Read the model definition and answer for the solid it produces. Units are mm, in the model's axes. A direction names the side the tool comes from. Coordinates: 2 decimals unless noted, no trailing zeros. Order: outer loops, then holes, each group sorted by start corner. A loop starts at its lowest first (then second) coordinate and runs counter-clockwise, first axis right, second up. Notation, with made-up numbers: (13, 6.5) -> (65, 6.5) arc R18 cw to (65, 11.5) -> close; hole circle Ø3 at (86.25, 19.25). An arc over 180 degrees is marked (long way). Use CSV: the item, a comma, the result in double quotes.
```python
from build123d import *

# Parameters (mm, degrees)
EXTRUDE_1_DEPTH          = 20
SKETCH_2_R               = 4.5
CUT_EXTRUDE_2_DEPTH      = 95.074438611
MIRROR_2_COPY_1_SKETCH_R = 4.5
MIRROR_2_COPY_1_DEPTH    = 95.074438611
SKETCH_3_R               = 55
CUT_EXTRUDE_3_DEPTH      = 95.074438611
EXTRUDE_2_DEPTH          = 20
SKETCH_6_R               = 5
CUT_EXTRUDE_4_DEPTH      = 143.828568571
SKETCH_1312_R            = 2.5
CUT_EXTRUDE_5_DEPTH      = 10


with BuildPart() as part:
    # 草圖1 → 填料-伸長1 (new body)
    with BuildSketch(Plane.XY):
        with BuildLine():
            Line((-55, 65), (55, 65))
            ThreePointArc((55, 65), (62.071067812, 62.071067812), (65, 55))
            Line((65, 55), (65, -65))
            Line((65, -65), (-65, -65))
            Line((-65, -65), (-65, 55))
            ThreePointArc((-65, 55), (-62.071067812, 62.071067812), (-55, 65))
        make_face()
    extrude(amount=EXTRUDE_1_DEPTH)

    # 草圖2 → 除料-伸長2 (cut, through all)
    with BuildSketch(Plane.XY):
        with Locations((51.25, 51.25)):
            Circle(SKETCH_2_R)
    cut_extrude_2 = extrude(amount=CUT_EXTRUDE_2_DEPTH, mode=Mode.SUBTRACT)

    # 鏡射1: 除料-伸長2 across plane
    add(cut_extrude_2.mirror(Plane(origin=(0, 0, 0), x_dir=(0, 0, 1), z_dir=(1, 0, 0))), mode=Mode.SUBTRACT)

    # 鏡射2: 除料-伸長2 across plane
    add(cut_extrude_2.mirror(Plane.ZX), mode=Mode.SUBTRACT)

    # 鏡射2 copy 1 sketch → 鏡射2 copy 1 (cut, through all)
    with BuildSketch(Plane(origin=(0, 0, 0), x_dir=(-1, 0, 0), z_dir=(0, 0, 1))):
        with Locations((51.25, 51.25)):
            Circle(MIRROR_2_COPY_1_SKETCH_R)
    extrude(amount=MIRROR_2_COPY_1_DEPTH, mode=Mode.SUBTRACT)

    # 草圖3 → 除料-伸長3 (cut, through all)
    with BuildSketch(Plane.XY):
        Circle(SKETCH_3_R)
    extrude(amount=CUT_EXTRUDE_3_DEPTH, mode=Mode.SUBTRACT)

    # 草圖5 → 填料-伸長2 (add)
    with BuildSketch(Plane.XY):
        with BuildLine():
            Line((65, -65), (100, -65))
            Line((100, -65), (100, -40))
            ThreePointArc((100, -40), (98.535533906, -36.464466094), (95, -35))
            Line((95, -35), (65, -35))
            Line((65, -35), (65, -65))
        make_face()
    extrude_2 = extrude(amount=EXTRUDE_2_DEPTH)

    # 草圖6 → 除料-伸長4 (cut, through all)
    with BuildSketch(Plane(origin=(0, -35, 0), x_dir=(1, 0, 0), z_dir=(0, 1, 0))):
        with Locations(Location((80, -10, 0), (0, 0, 180))):
            Circle(SKETCH_6_R)
    cut_extrude_4 = extrude(amount=-CUT_EXTRUDE_4_DEPTH, mode=Mode.SUBTRACT)

    # 鏡射3: 填料-伸長2 across plane
    add(extrude_2.mirror(Plane(origin=(0, 0, 0), x_dir=(0, 0, 1), z_dir=(1, 0, 0))))

    # 鏡射4: 除料-伸長4 across plane
    add(cut_extrude_4.mirror(Plane(origin=(0, 0, 0), x_dir=(0, 0, 1), z_dir=(1, 0, 0))), mode=Mode.SUBTRACT)

    # Sketch 1312 → 除料-伸長5 (cut)
    with BuildSketch(Plane(origin=(0, 0, 0), x_dir=(-1, 0, 0), z_dir=(0, 0, -1))):
        with Locations((59.84, -48.46)):
            Circle(SKETCH_1312_R)
        with Locations((-59.84, 48.46)):
            Circle(SKETCH_1312_R)
    extrude(amount=-CUT_EXTRUDE_5_DEPTH, mode=Mode.SUBTRACT)


solid = part.part
```
Item 1: Find section B-B, the plane z = 3. Give the vertices of the cut face in (x, y).
Return value:
outline,"(-100, -65) -> (100, -65) -> (100, -40) arc R5 ccw to (95, -35) -> (65, -35) -> (65, 55) arc R10 ccw to (55, 65) -> (-55, 65) arc R10 ccw to (-65, 55) -> (-65, -35) -> (-95, -35) arc R5 ccw to (-100, -40) -> close; hole circle Ø5 at (-59.84, -48.46); hole circle Ø9 at (-51.25, -51.25); hole circle Ø9 at (-51.25, 51.25); hole circle Ø110 at (0, 0); hole circle Ø9 at (51.25, -51.25); hole circle Ø9 at (51.25, 51.25); hole circle Ø5 at (59.84, 48.46)"
Item 2: A tool of negligible diameter and unlimited length cuts with its end or side. For faces 4 (the flat face through (65, 11, 10)), 5 (the cylindrical face through (-62.15, -49.42, 4.93)), 6 (the flat face through (-84, -35, 5)), 7 (the cylindrical face through (-11.923, -53.692, 9.86)), 8 (the cylindrical face through (-75.381, -49.79, 8.085)), from which of +Z, -Z, +X, -X, +Y, -Y can it reach the whole face along a straight path? Write none if from no direction.
Return value:
face 4,"+Z, -Z, +X, +Y"
face 5,"-Z"
face 6,"+Z, -Z, -X, +Y"
face 7,"+Z, -Z"
face 8,"+Y, -Y"
Item 3: Each of these flat-tipped pins is pushed along its axis until it touches: P1, Ø10, axis at y = -10, z = 4.5, coming from the -X side; P2, Ø14.5, axis at x = -51.25, y = 51.25, coming from the -Z side; P3, Ø3, axis at x = -59.84, y = -48.46, coming from the -Z side; P4, Ø4, axis at y = 6.5, z = 15.5, coming from the +X side. Where does it stop, or does it pass through?
Return value:
P1,"stops at x = -65"
P2,"stops at z = 0"
P3,"stops at z = 10"
P4,"stops at x = 65"
Item 4: Find section A-A, the plane x = 0. Give the vertices of the cut face in (y, z), then the cut area to 3 significant figures.
Return value:
outline,"(-65, 0) -> (-55, 0) -> (-55, 20) -> (-65, 20) -> close; (55, 0) -> (65, 0) -> (65, 20) -> (55, 20) -> close"
area,"400 mm^2"
Item 5: Find section C-C, the plane z = 13. Give the vertices of the cut face in (x, y), then the cut area to 3 significant figures.
Return value:
outline,"(-100, -65) -> (-84, -65) -> (-84, -35) -> (-95, -35) arc R5 ccw to (-100, -40) -> close; (-76, -65) -> (76, -65) -> (76, -35) -> (65, -35) -> (65, 55) arc R10 ccw to (55, 65) -> (-55, 65) arc R10 ccw to (-65, 55) -> (-65, -35) -> (-76, -35) -> close; (84, -65) -> (100, -65) -> (100, -40) arc R5 ccw to (95, -35) -> (84, -35) -> close; hole circle Ø9 at (-51.25, -51.25); hole circle Ø9 at (-51.25, 51.25); hole circle Ø110 at (0, 0); hole circle Ø9 at (51.25, -51.25); hole circle Ø9 at (51.25, 51.25)"
area,"8,710 mm^2"
Item 6: Straight lines are drawn through the part: line 1 along Y through (x, z) = (0, 9); line 2 along X through (y, z) = (10.5, 17); line 3 along X through (y, z) = (33.5, 1.75). For each, find the intervals that lie inside material, in ascending order.
Return value:
line 1,"y = -65 to -55, 55 to 65"
line 2,"x = -65 to -53.99, 53.99 to 65"
line 3,"x = -65 to -43.62, 43.62 to 65"
Item 7: The mould has two halves that part along X. Classify faces 1 (the cylindrical face through (-99, -37, 10)), 2 (the cylindrical face through (61.99, 62.15, 9.86)), 3 (the cylindrical face through (62.338, 48.57, 4.93)): +X half, -X half, draft (parallel to the pull), parting line (faces both ways), or undercut.
Return value:
face 1,"-X half"
face 2,"+X half"
face 3,"undercut"
Item 8: Find section D-D, the plane x = -51.25. Give the vertices of the cut face in (y, z), then the cut area to 3 significant figures.
Return value:
outline,"(-65, 0) -> (-55.75, 0) -> (-55.75, 20) -> (-65, 20) -> close; (-46.75, 0) -> (-19.96, 0) -> (-19.96, 20) -> (-46.75, 20) -> close; (19.96, 0) -> (46.75, 0) -> (46.75, 20) -> (19.96, 20) -> close; (55.75, 0) -> (65, 0) -> (65, 20) -> (55.75, 20) -> close"
area,"1,440 mm^2"
